Can you work these out from the model? Positions are in its coordinate system, mm. Face numbers are marked on the shaded views. A direction names the side the tool comes from. Give positions to 0.01 mm unless a question says otherwise; leave off trailing zeros. Write each loop counter-clockwise with the first axis right and the second up, starting at its lowest first coordinate (ties: lowest second). Pieces come first, ordered by that corner, then holes.
```python
from build123d import *

# Parameters (mm, degrees)
SKETCH_1_W          = 19
SKETCH_1_H          = 26
SKETCH_1_R          = 3.05
SKETCH_1_R_2        = 1.05
SKETCH_1_R_3        = 2.1
SKETCH_1_R_4        = 2.55
EXTRUDE_1_DEPTH     = 2.5
CUT_EXTRUDE_START   = 2.5
SKETCH_1_3_R        = 1
CUT_EXTRUDE_2_DEPTH = 1.5
SKETCH_1_4_R        = 0.8
CUT_EXTRUDE_3_DEPTH = 1.5
SKETCH_2_R          = 2.5
SKETCH_2_R_2        = 2
EXTRUDE_2_DEPTH     = 14.5
CUT_EXTRUDE_START_2 = 14.5
SKETCH_2_4_R        = 0.3
CUT_EXTRUDE_6_DEPTH = 1.5
SKETCH_4_R          = 1
CUT_EXTRUDE_7_DEPTH = 1.5
SKETCH_4_3_R        = 0.7
CUT_EXTRUDE_8_DEPTH = 26.124689053
SKETCH_3_R          = 0.3
CUT_EXTRUDE_9_DEPTH = 1.5


with BuildPart() as part:
    # 草图1 → 凸台-拉伸1 (new body)
    with BuildSketch(Plane(origin=(0, 0, 0), x_dir=(1, 0, 0), z_dir=(0, 1, 0))):
        with Locations((4.5, -2)):
            Rectangle(SKETCH_1_W, SKETCH_1_H)
        with Locations(Location((0, 0, 0), (0, 0, 270))):
            Circle(SKETCH_1_R, mode=Mode.SUBTRACT)
        with Locations(Location((8.107149516, 2.554237014, 0), (0, 0, 270))):
            Circle(SKETCH_1_R_2, mode=Mode.SUBTRACT)
        with Locations(Location((3.9, 6.4, 0), (0, 0, 270))):
            Circle(SKETCH_1_R, mode=Mode.SUBTRACT)
        with Locations(Location((1, -10, 0), (0, 0, 270))):
            Circle(SKETCH_1_R_3, mode=Mode.SUBTRACT)
        with Locations(Location((6.694056557, -4.380594344, 0), (0, 0, 270))):
            Circle(SKETCH_1_R_4, mode=Mode.SUBTRACT)
    extrude(amount=EXTRUDE_1_DEPTH)

    # 草图1<3> → 切除-拉伸2 (cut)
    with BuildSketch(Plane(origin=(0, 0, 0), x_dir=(1, 0, 0), z_dir=(0, 1, 0)).offset(CUT_EXTRUDE_START)):
        with Locations(Location((-3.5, -10, 0), (0, 0, 90))):
            Circle(SKETCH_1_3_R)
        with Locations(Location((5.5, -10, 0), (0, 0, 90))):
            Circle(SKETCH_1_3_R)
    extrude(amount=-CUT_EXTRUDE_2_DEPTH, mode=Mode.SUBTRACT)

    # 草图1<4> → 切除-拉伸3 (cut)
    with BuildSketch(Plane(origin=(0, 0, 0), x_dir=(1, 0, 0), z_dir=(0, 1, 0))):
        with Locations(Location((-3.5, -10, 0), (0, 0, 90))):
            Circle(SKETCH_1_4_R)
        with Locations(Location((5.5, -10, 0), (0, 0, 90))):
            Circle(SKETCH_1_4_R)
    extrude(amount=CUT_EXTRUDE_3_DEPTH, mode=Mode.SUBTRACT)

    # 草图2 → 凸台-拉伸2 (add)
    with BuildSketch(Plane(origin=(0, 2.5, 0), x_dir=(1, 0, 0), z_dir=(0, 1, 0))):
        with Locations(Location((11.5, -12.5, 0), (0, 0, 270))):
            Circle(SKETCH_2_R)
        with Locations(Location((-3, -6, 0), (0, 0, 180))):
            Circle(SKETCH_2_R_2)
    extrude(amount=EXTRUDE_2_DEPTH)

    # 草图2<4> → 切除-拉伸6 (cut)
    with BuildSketch(Plane(origin=(0, 2.5, 0), x_dir=(1, 0, 0), z_dir=(0, 1, 0)).offset(CUT_EXTRUDE_START_2)):
        with Locations(Location((11.5, -12.5, 0), (0, 0, 270))):
            Circle(SKETCH_2_4_R)
        with Locations(Location((-3, -6, 0), (0, 0, 270))):
            Circle(SKETCH_2_4_R)
    extrude(amount=-CUT_EXTRUDE_6_DEPTH, mode=Mode.SUBTRACT)

    # 草图4 → 切除-拉伸7 (cut)
    with BuildSketch(Plane(origin=(0, 2.5, 0), x_dir=(1, 0, 0), z_dir=(0, 1, 0))):
        with Locations(Location((12, 9, 0), (0, 0, 270))):
            Circle(SKETCH_4_R)
        with Locations(Location((-3, 9, 0), (0, 0, 270))):
            Circle(SKETCH_4_R)
        with Locations(Location((12, -3, 0), (0, 0, 270))):
            Circle(SKETCH_4_R)
    extrude(amount=-CUT_EXTRUDE_7_DEPTH, mode=Mode.SUBTRACT)

    # 草图4<3> → 切除-拉伸8 (cut, through all)
    with BuildSketch(Plane(origin=(0, 2.5, 0), x_dir=(1, 0, 0), z_dir=(0, 1, 0))):
        with Locations(Location((12, 9, 0), (0, 0, 270))):
            Circle(SKETCH_4_3_R)
        with Locations(Location((-3, 9, 0), (0, 0, 270))):
            Circle(SKETCH_4_3_R)
        with Locations(Location((12, -3, 0), (0, 0, 270))):
            Circle(SKETCH_4_3_R)
    extrude(amount=-CUT_EXTRUDE_8_DEPTH, mode=Mode.SUBTRACT)

    # 草图3 → 切除-拉伸9 (cut)
    with BuildSketch(Plane.XY.offset(-11)):
        with Locations((-1, 1.25)):
            Circle(SKETCH_3_R)
        with Locations((4, 1.25)):
            Circle(SKETCH_3_R)
    extrude(amount=CUT_EXTRUDE_9_DEPTH, mode=Mode.SUBTRACT)


solid = part.part
```
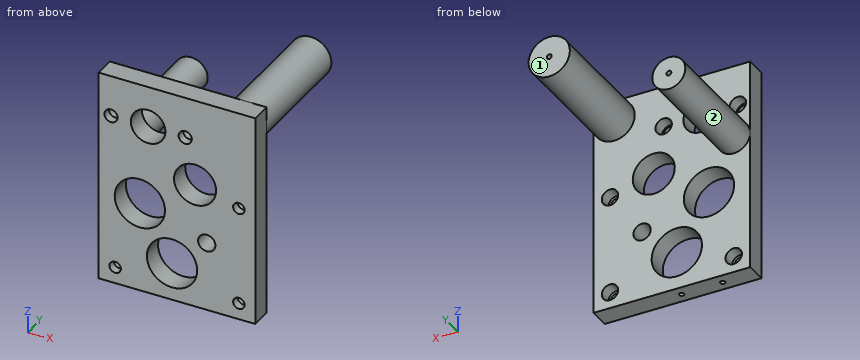
1) For the marked faces 1 and 2, which set-ups out of +Z, -Z, +X, -X, +Y, -Y let a thin tool reach every point of the face, with its end or its side?
Values follow:
face 1: +Z, -Z, +X, -X, +Y
face 2: +Y
2) Please list where these lines run through material, in increasing order: L1, parallel to X at y = 1.65, z = 10; L2, parallel to X at y = 0.65, z = 0; L3, parallel to Z at x = 1.75, y = 1.25.
Values follow:
L1: x = -5 to -4.5, -2.5 to -1.1, 3.1 to 4.5, 6.5 to 14
L2: x = -5 to -3.05, 3.05 to 14
L3: z = -11 to -8.56, -4.24 to -2.5, 2.5 to 8.04, 11.96 to 15
3) Suppose I cut it at D-D on z = -9. Write out the boundary of the cut face in (x, y).
Values follow:
outline: (-5, 0) - (-3.7, 0) - (-3.7, 1) - (-4, 1) - (-4, 2.5) - (-5, 2.5) - close; (-2.3, 0) - (2.31, 0) - (2.31, 2.5) - (-2, 2.5) - (-2, 1) - (-2.3, 1) - close; (5.49, 0) - (11.3, 0) - (11.3, 1) - (11, 1) - (11, 2.5) - (5.49, 2.5) - close; (12.7, 0) - (14, 0) - (14, 2.5) - (13, 2.5) - (13, 1) - (12.7, 1) - close
4) Suppose I cut it at A-A on z = 11.5. Write out the boundary of the cut face in (x, y), plus the area to 3 significant figures.
Values follow:
outline: (-5, 0) - (-0.47, 0) - (-0.47, 2.5) - (-5, 2.5) - close; (2.47, 0) - (14, 0) - (14, 2.5) - (13.79, 2.5) - (13.79, 17) - (9.21, 17) - (9.21, 2.5) - (2.47, 2.5) - close
area: 107 mm2
5) For pin 1 Ø8 at (y, z) = (14, -0.5) entering from +X; pin 2 Ø5 at (y, z) = (11, 2.5) entering from +X; pin 3 Ø10 at (y, z) = (9.5, 5) entering from -X; pin 4 Ø1.8 at (x, z) = (12, 3) entering from +Y, each with a flat end and sliding along its axis, tell me the tip position at first contact or that it passes through.
Values follow:
pin 1: passes through
pin 2: stops at x = -1.27
pin 3: stops at x = -5
pin 4: stops at y = 1
6) Suppose I cut it at C-C on y = 15. Write out the boundary of the cut face in (x, z).
Values follow:
outline: circle Ø4 at (-3, 6); circle Ø5 at (11.5, 12.5)
7) Suppose I cut it at B-B on x = 5.5. Write out the boundary of the cut face in (y, z), plus the area to 3 significant figures.
Values follow:
outline: (0, -11) - (2.5, -11) - (2.5, -9) - (0, -9) - close; (0, -3.8) - (2.5, -3.8) - (2.5, 2.13) - (0, 2.13) - close; (0, 6.63) - (2.5, 6.63) - (2.5, 9) - (1, 9) - (1, 9.2) - (0, 9.2) - close; (0, 10.8) - (1, 10.8) - (1, 11) - (2.5, 11) - (2.5, 15) - (0, 15) - close
area: 36.2 mm2
